Here's how the part is built. I have some questions about the finished solid (model axes, mm). A direction names the side the tool comes from. Give positions to 0.01 mm unless a question says otherwise; leave off trailing zeros. Loops run counter-clockwise (first coordinate to the right, second up) from the corner with the lowest first, then second, coordinate; pieces in that order, holes last. Notation, with made-up numbers: (11, 29) - (20, 29) arc R14 ccw to (20, 40) - close; hole circle Ø6 at (-34.5, -15). An arc over 180 degrees is marked (long way). One line per item, written item: value. Start each with the question number.
```python
from build123d import *

# Parameters (mm, degrees)
F0_R     = 31.496
F1_DEPTH = 63.5
F2_DEPTH = 63.5
F3_DEPTH = 63.5


with BuildPart() as f1:
    # F0 (on Front) → F1 (new body)
    with BuildSketch(Plane.XZ):
        Circle(F0_R)
        with BuildLine():
            ThreePointArc((26.416, 0), (26.1371583003, -3.8280559015), (25.306519989, -7.5752955087))
            ThreePointArc((25.306519989, -7.5752955087), (22.8769270664, -13.208), (19.2136583462, -18.1284414375))
            ThreePointArc((19.2136583462, -18.1284414375), (0, -26.416), (-19.2136583462, -18.1284414375))
            ThreePointArc((-19.2136583462, -18.1284414375), (-22.9056297562, -13.1581602617), (-25.3392663756, -7.4650274981))
            ThreePointArc((-25.3392663756, -7.4650274981), (-22.8481158541, 13.2577772615), (-6.0928613417, 25.7037370176))
            ThreePointArc((-6.0928613417, 25.7037370176), (-4.8286381359, 25.9709320155), (-3.5528613417, 26.175985794))
            ThreePointArc((-3.5528613417, 26.175985794), (17.3774663113, 19.8954447199), (26.416, 0))
        make_face(mode=Mode.SUBTRACT)
    extrude(amount=F1_DEPTH)



with BuildPart() as f2:
    # F0 (on Front) → F2 (new body)
    with BuildSketch(Plane.XZ):
        with BuildLine():
            ThreePointArc((2.8770503286, -5.3743648375), (5.2297091125, -3.1323088287), (6.096, 0))
            ThreePointArc((6.096, 0), (5.3275135744, 2.9629065315), (3.2158113142, 5.1787810913))
            ThreePointArc((3.2158113142, 5.1787810913), (0.013272421, 6.0959855514), (-3.1932300386, 5.1927351098))
            ThreePointArc((-3.1932300386, 5.1927351098), (-3.3751638093, 5.0763653592), (-3.5528613417, 4.9536241568))
            ThreePointArc((-3.5528613417, 4.9536241568), (-5.3777045607, 2.8708029639), (-6.0928613417, 0.1955931265))
            ThreePointArc((-6.0928613417, 0.1955931265), (-5.2792932077, -3.0479959361), (-2.8770503286, -5.3743648375))
            ThreePointArc((-2.8770503286, -5.3743648375), (0, -6.096), (2.8770503286, -5.3743648375))
        make_face()
        with BuildLine():
            ThreePointArc((2.4892, 3.0502216903), (3.5566802921, 1.6881926134), (3.937, 0))
            ThreePointArc((3.937, 0), (3.5566802921, -1.6881926134), (2.4892, -3.0502216903))
            ThreePointArc((2.4892, -3.0502216903), (0.0964538394, -3.9358182957), (-2.3368, -3.1684909279))
            ThreePointArc((-2.3368, -3.1684909279), (-3.937, 0), (-2.3368, 3.1684909279))
            ThreePointArc((-2.3368, 3.1684909279), (0.0964538394, 3.9358182957), (2.4892, 3.0502216903))
        make_face(mode=Mode.SUBTRACT)
        with BuildLine():
            Line((-2.3368, -3.1684909279), (-2.3368, 3.1684909279))
            ThreePointArc((-2.3368, 3.1684909279), (-3.937, 0), (-2.3368, -3.1684909279))
        make_face()
        with BuildLine():
            ThreePointArc((2.4892, -3.0502216903), (3.5566802921, -1.6881926134), (3.937, 0))
            ThreePointArc((3.937, 0), (3.5566802921, 1.6881926134), (2.4892, 3.0502216903))
            Line((2.4892, 3.0502216903), (2.4892, -3.0502216903))
        make_face()
    extrude(amount=F2_DEPTH)


with BuildPart() as f1_1:
    add(f1.part)

    add(f2.part)  # F3 merges F2
    # F0 (on Front) → F3 (join)
    with BuildSketch(Plane.XZ):
        with BuildLine():
            Line((0, -7.0354306192), (2.8770503286, -5.3743648375))
            ThreePointArc((2.8770503286, -5.3743648375), (0, -6.096), (-2.8770503286, -5.3743648375))
            Line((-2.8770503286, -5.3743648375), (0, -7.0354306192))
        make_face()
        with BuildLine():
            Line((0, -7.0354306192), (-2.8770503286, -5.3743648375))
            ThreePointArc((-2.8770503286, -5.3743648375), (-5.2792932077, -3.0479959361), (-6.0928613417, 0.1955931265))
            Line((-6.0928613417, 0.1955931265), (-6.0928613417, 3.5354252361))
            Line((-6.0928613417, 3.5354252361), (-25.3392663756, -7.4650274981))
            ThreePointArc((-25.3392663756, -7.4650274981), (-22.9056297562, -13.1581602617), (-19.2136583462, -18.1284414375))
            Line((-19.2136583462, -18.1284414375), (0, -7.0354306192))
        make_face()
        with BuildLine():
            ThreePointArc((3.2158113142, 5.1787810913), (5.3275135744, 2.9629065315), (6.096, 0))
            ThreePointArc((6.096, 0), (5.2297091125, -3.1323088287), (2.8770503286, -5.3743648375))
            Line((2.8770503286, -5.3743648375), (0, -7.0354306192))
            Line((0, -7.0354306192), (19.2136583462, -18.1284414375))
            ThreePointArc((19.2136583462, -18.1284414375), (22.8769270664, -13.208), (25.306519989, -7.5752955087))
            Line((25.306519989, -7.5752955087), (3.2158113142, 5.1787810913))
        make_face()
        with BuildLine():
            ThreePointArc((-6.0928613417, 0.1955931265), (-5.3777045607, 2.8708029639), (-3.5528613417, 4.9536241568))
            Line((-3.5528613417, 4.9536241568), (-3.5528613417, 4.9871846631))
            Line((-3.5528613417, 4.9871846631), (-6.0928613417, 3.5354252361))
            Line((-6.0928613417, 3.5354252361), (-6.0928613417, 0.1955931265))
        make_face()
        with BuildLine():
            Line((-6.0928613417, 3.5354252361), (-3.5528613417, 4.9871846631))
            Line((-3.5528613417, 4.9871846631), (-3.5528613417, 26.175985794))
            ThreePointArc((-3.5528613417, 26.175985794), (-4.8286381359, 25.9709320155), (-6.0928613417, 25.7037370176))
            Line((-6.0928613417, 25.7037370176), (-6.0928613417, 3.5354252361))
        make_face()
        with BuildLine():
            Line((-25.3392663756, -7.4650274981), (-6.0928613417, 3.5354252361))
            Line((-6.0928613417, 3.5354252361), (-6.0928613417, 25.7037370176))
            ThreePointArc((-6.0928613417, 25.7037370176), (-22.8481158541, 13.2577772615), (-25.3392663756, -7.4650274981))
        make_face()
        with BuildLine():
            ThreePointArc((-3.1932300386, 5.1927351098), (0.013272421, 6.0959855514), (3.2158113142, 5.1787810913))
            Line((3.2158113142, 5.1787810913), (25.306519989, -7.5752955087))
            ThreePointArc((25.306519989, -7.5752955087), (26.1371583003, -3.8280559015), (26.416, 0))
            ThreePointArc((26.416, 0), (17.3774663113, 19.8954447199), (-3.5528613417, 26.175985794))
            Line((-3.5528613417, 26.175985794), (-3.5528613417, 4.9871846631))
            Line((-3.5528613417, 4.9871846631), (-3.1932300386, 5.1927351098))
        make_face()
        with BuildLine():
            ThreePointArc((-3.5528613417, 4.9536241568), (-3.3751638093, 5.0763653592), (-3.1932300386, 5.1927351098))
            Line((-3.1932300386, 5.1927351098), (-3.5528613417, 4.9871846631))
            Line((-3.5528613417, 4.9871846631), (-3.5528613417, 4.9536241568))
        make_face()
        with BuildLine():
            Line((19.2136583462, -18.1284414375), (0, -7.0354306192))
            Line((0, -7.0354306192), (-19.2136583462, -18.1284414375))
            ThreePointArc((-19.2136583462, -18.1284414375), (0, -26.416), (19.2136583462, -18.1284414375))
        make_face()
    extrude(amount=F3_DEPTH)


solid = f1_1.part
```
(1) For faces 4 (the face through (0.06, -31.306, 3.937)), 5 (the face through (0, 0, -7)), which set-ups out of +Z, -Z, +X, -X, +Y, -Y let a thin tool reach every point of the face, with its end or its side?
(2) If we section it at B-B on x = 0: List the corners of the cut face in (y, z) for me, plus the area to 3 significant figures.
(3) Will these pins go through, and if not, where does the flat tip stop? pin 1 (1 mm diameter, centred on y = -44.5, z = 13.5, fed in from +X); pin 2 (6 mm diameter, centred on y = -10.5, z = -8.5, fed in from -X); pin 3 (2 mm diameter, centred on x = -0.5, y = -18, fed in from -Z).
(4) If we mould it in two halves opening along X, with no side actions, what happens to faces 1 (the face through (-6.828, -31.306, -30.747)), 2 (the face through (0, -63.5, -7)), 3 (the face through (0.133, -31.306, -3.935))? For each: pulls with the +X half, pulls with the -X half, needs draft (parallel to the pull), parting line crosses it, or undercut.
(5) If we section it at A-A on z = 0: List the corners of the cut face in (x, y) for me, plus the area to 3 significant figures.
(6) If we section it at D-D on x = 25: List the corners of the cut face in (y, z) for me.
(7) Please list where these lines run through material, in increasing order: probe 1 along X at (y, z) = (-54, 1); probe 2 along Z at (x, y) = (-10.5, -44); probe 3 along X at (y, z) = (-11, -7). Write a range as from..to.
(8) If we section it at C-C on y = -52: List the corners of the cut face in (x, z) for me, plus the area to 3 significant figures.
Found:
1. face 4: +Y, -Y
1. face 5: +Z, -Z, +X, -X, +Y
2. outline: (-63.5, -31.5) - (0, -31.5) - (0, -3.94) - (-63.5, -3.94) - close; (-63.5, 3.94) - (0, 3.94) - (0, 31.5) - (-63.5, 31.5) - close
2. area: 3,500 mm^2
3. pin 1: x = 28.69
3. pin 2: x = -31.01
3. pin 3: z = -31.5
4. face 1: parting line crosses it
4. face 2: needs draft
4. face 3: undercut
5. outline: (-31.5, -63.5) - (-2.34, -63.5) - (-2.34, 0) - (-31.5, 0) - close; (2.49, -63.5) - (31.5, -63.5) - (31.5, 0) - (2.49, 0) - close
5. area: 3,690 mm^2
6. outline: (-63.5, -19.16) - (0, -19.16) - (0, 19.16) - (-63.5, 19.16) - close
7. probe 1: -31.48..-2.34, 2.49..31.48
7. probe 2: -29.69..29.69
7. probe 3: -30.71..30.71
8. outline: circle Ø62.99 at (0, 0); hole (-2.34, -3.17) arc R3.94 ccw to (2.49, -3.05) - (2.49, 3.05) arc R3.94 ccw to (-2.34, 3.17) - close
8. area: 3,080 mm^2
